Verification items for this drawing (mm, ordinates from the low corner). A direction names the side the tool comes from. Give positions to 0.01 mm unless a question says otherwise; leave off trailing zeros. Loops run counter-clockwise (first coordinate to the right, second up) from the corner with the lowest first, then second, coordinate; pieces in that order, holes last. Notation, with made-up numbers: (-18, 52) -> (30, 52) arc R23 ccw to (30, 80) -> close; hole circle Ø9 at (38.25, 55.25). An arc over 180 degrees is marked (long way). Answer as a JSON object with one key per item and string values.
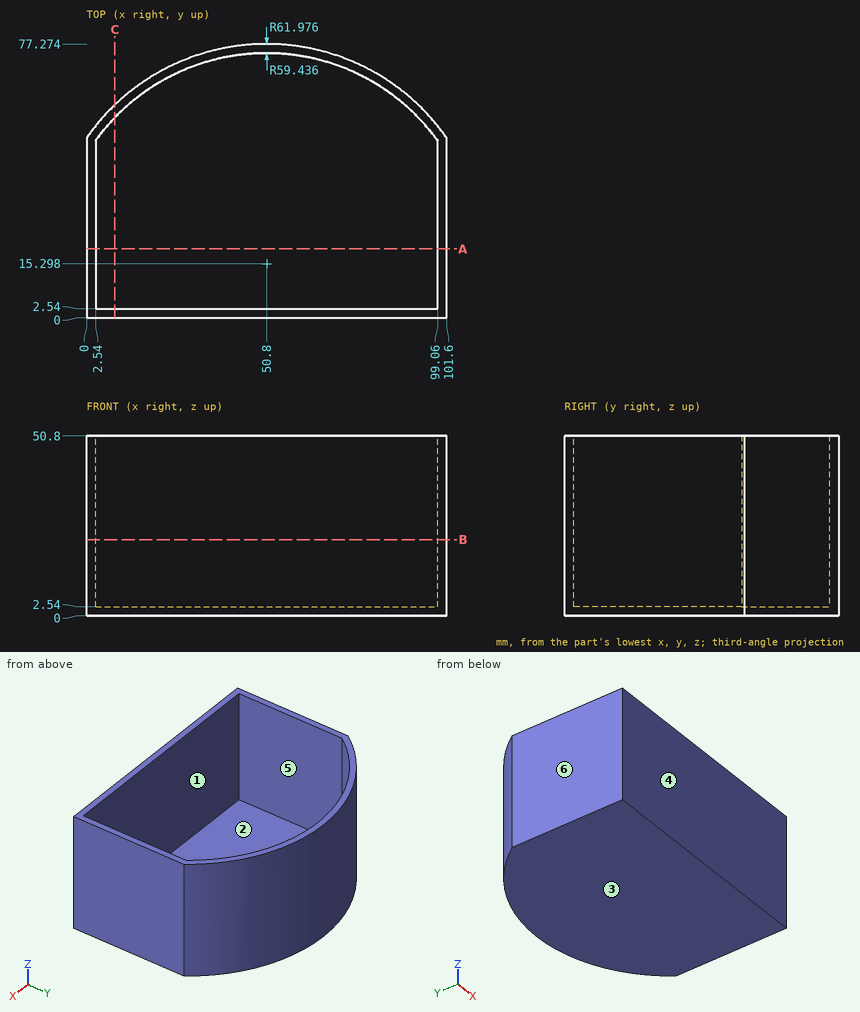
1) Tool access check on the marked faces 5 and 6. Record the directions out of +Z, -Z, +X, -X, +Y, -Y that give a thin tool (end or side, any length) a straight path to the whole face; none if there is none.
Geometry check:
{"face 5": "+Z", "face 6": "+Z, -Z, -X, +Y, -Y"}
2) Section check C-C on x = 8. Record the cut outline in (y, z), plus the area to 3 significant figures.
Geometry check:
{"outline": "(0, 0) -> (60.12, 0) -> (60.12, 50.8) -> (56.54, 50.8) -> (56.54, 2.54) -> (2.54, 2.54) -> (2.54, 50.8) -> (0, 50.8) -> close", "area": "448 mm2"}
3) Draft check along Y on the marked faces 1, 2, 3 and 4. Enter one of: pulls with the +Y half, pulls with the -Y half, needs draft (parallel to the pull), parting line crosses it, or undercut.
Geometry check:
{"face 1": "undercut", "face 2": "undercut", "face 3": "needs draft", "face 4": "pulls with the -Y half"}
4) Depth check by flat-ended pin: P1, Ø6, axis at x = 43, z = 22.5, coming from the +Y side; P2, Ø4, axis at y = 68, z = 36.5, coming from the -X side; P3, Ø4, axis at x = 78.5, y = 38.5, coming from the +Z side. Enter the tip coordinate at first touch or a pass-through.
Geometry check:
{"P1": "stops at y = 77.09", "P2": "stops at x = 15.16", "P3": "stops at z = 2.54"}
5) Section check B-B on z = 21.5. Record the cut outline in (x, y).
Geometry check:
{"outline": "(0, 0) -> (101.6, 0) -> (101.6, 50.8) arc R61.98 ccw to (0, 50.8) -> close; hole (2.54, 2.54) -> (99.06, 2.54) -> (99.06, 49.99) arc R59.44 ccw to (2.54, 49.99) -> close"}
6) Material ranges on line 1 along X through (y, z) = (35.5, 5); line 2 along Y through (x, z) = (49.5, 5); line 3 along Z through (x, y) = (23.5, 23), recorded low to high. Write a range as from..to.
Geometry check:
{"line 1": "x = 0..2.54, 99.06..101.6", "line 2": "y = 0..2.54, 74.72..77.26", "line 3": "z = 0..2.54"}
7) Section check A-A on y = 19.5. Record the cut outline in (x, z), plus the area to 3 significant figures.
Geometry check:
{"outline": "(0, 0) -> (101.6, 0) -> (101.6, 50.8) -> (99.06, 50.8) -> (99.06, 2.54) -> (2.54, 2.54) -> (2.54, 50.8) -> (0, 50.8) -> close", "area": "503 mm2"}
